CAD build for the part. Positions are in the model's coordinates, mm. A direction names the side the tool comes from. Coordinates: 2 decimals unless noted, no trailing zeros. Write each loop counter-clockwise with the first axis right and the second up, starting at its lowest first coordinate (ties: lowest second). Pieces come first, ordered by that corner, then holes. Notation, with made-up numbers: M -31.75,-6 L 27.25,-6 A15 ccw 27.25,8 Z; hole C 45,33.25 d10. An arc over 180 degrees is marked long. Put each result on its own line as item: value. Start each with the question number.
```python
from build123d import *

# Parameters (mm, degrees)
SKETCH1_R           = 15.94
SKETCH1_R_2         = 14.94
BOSS_EXTRUDE1_DEPTH = 7
SKETCH1_3_R         = 20.5
SKETCH1_3_R_2       = 15.94
BOSS_EXTRUDE2_DEPTH = 5
CHAMFER1_SIZE       = 2
SKETCH2_W           = 8
SKETCH2_H           = 2.482498026
CUT_EXTRUDE1_DEPTH  = 13


with BuildPart() as part:
    # Sketch1 → Boss-Extrude1 (new body)
    with BuildSketch(Plane.XY):
        Circle(SKETCH1_R)
        Circle(SKETCH1_R_2, mode=Mode.SUBTRACT)
    extrude(amount=BOSS_EXTRUDE1_DEPTH)

    # Sketch1<3> → Boss-Extrude2 (add)
    with BuildSketch(Plane.XY):
        Circle(SKETCH1_3_R)
        Circle(SKETCH1_3_R_2, mode=Mode.SUBTRACT)
    extrude(amount=BOSS_EXTRUDE2_DEPTH)

    # Chamfer1
    chamfer1_edges = [part.edges().sort_by_distance(p)[0] for p in [
        (-20.5, 0, 5),
    ]]
    chamfer(chamfer1_edges, length=CHAMFER1_SIZE)

    # Sketch2 → Cut-Extrude1 (cut)
    with BuildSketch(Plane(origin=(20.5, 0, 0), x_dir=(0, 0, -1), z_dir=(1, 0, 0))):
        with Locations((-3, 0)):
            Rectangle(SKETCH2_W, SKETCH2_H)
    extrude(amount=-CUT_EXTRUDE1_DEPTH, mode=Mode.SUBTRACT)


solid = part.part
```
(1) Drill centre lines: line 1 (X direction, y = 11.5, z = 0.5); line 2 (Z direction, x = -5, y = 15.5); line 3 (X direction, y = 5.5, z = 2.75). Where is each one in solid material? Low to high. Write a range as [from, to].
(2) Drop flat-ended pins along their axis: pin 1 (1 mm diameter, centred on y = 13, z = 4.5, fed in from -X); pin 2 (18 mm diameter, centred on x = 0, y = 0, fed in from +Z); pin 3 (4 mm diameter, centred on x = 11.5, z = 4.5, fed in from -Y); pin 4 (1.7 mm diameter, centred on x = 16.5, z = 4, fed in from -Y). Give the stop position or say it passes through.
(3) Two-plate mould, pull along X, no slides. Class faces 4 (the face through (-20.48, 0.88, 1.48)), 5 (the face through (-11, -11, 7)), 6 (the face through (-14.926, 0.64, 3.451)): +X half, -X half, draft (parallel to the pull), parting line (faces both ways), or undercut.
(4) Which spindle directions (+Z, -Z, +X, -X, +Y, -Y) get a long thin tool onto all of the face, cutting with end or side? Do faces 1 (the face through (17, -1.241, 3)), 2 (the face through (-15.925, 0.683, 5.986)), 3 (the face through (6, 14, 0)). Say none if no direction does.
(5) Slice it at A-A, the plane y = 0. Write the cut outline in (x, z), then the cut area to 3 significant figures.
(6) Slice it at C-C, the plane z = 2.25. Write the cut outline in (x, y), then the cut area to 3 significant figures.
(7) Slice it at B-B, the plane z = 5.5. Write the cut outline in (x, y), then the cut area to 3 significant figures.
Result set:
1. line 1: x = [-16.97, -9.54], [9.54, 16.97]
1. line 2: z = [0, 5]
1. line 3: x = [-19.75, -13.89], [13.89, 19.75]
2. pin 1: stops at x = -14.67
2. pin 2: passes through
2. pin 3: stops at y = -17.8
2. pin 4: stops at y = -12.31
3. face 4: parting line
3. face 5: draft
3. face 6: undercut
4. face 1: +Z, -Z, +X
4. face 2: +Z
4. face 3: -Z, +X, -X, +Y, -Y
5. outline: M -20.5,0 L -14.94,0 L -14.94,7 L -15.94,7 L -15.94,5 L -18.5,5 L -20.5,3 Z
5. area: 27.8 mm^2
6. outline: M 14.89,-1.24 A14.94 cw long 14.89,1.24 L 20.46,1.24 A20.5 ccw long 20.46,-1.24 Z
6. area: 605 mm^2
7. outline: M 14.89,-1.24 A14.94 cw long 14.89,1.24 L 15.89,1.24 A15.94 ccw long 15.89,-1.24 Z
7. area: 94.5 mm^2
